Source: CAD feature listing. Evaluate the final solid. Frame: model axes, mm. Face numbers are marked on the shaded views. A direction names the side the tool comes from. Round coordinates to 2 decimals unless told otherwise and drop trailing zeros. Write each loop counter-clockwise with the first axis right and the second up, starting at its lowest first coordinate (ties: lowest second). Pieces come first, ordered by that corner, then holes.
```python
from build123d import *

# Parameters (mm, degrees)
MAIN_BODY_DEPTH      = 15
HOLES_DEPTH          = 84.815273071
HEX_NUT_RECESS_DEPTH = 3


with BuildPart() as part:
    # Schizzo2 → Main Body (new, symmetric)
    with BuildSketch(Plane(origin=(0, 0, 0), x_dir=(1, 0, 0), z_dir=(0, 1, 0))):
        with BuildLine():
            Line((0, 0), (0, 20))
            Line((0, 20), (24.437059837, 20))
            Line((24.437059837, 20), (24.437059837, 10.75))
            Line((24.437059837, 10.75), (14.437059837, 10.75))
            ThreePointArc((14.437059837, 10.75), (5.5, 10), (14.437059837, 9.25))
            Line((14.437059837, 9.25), (80, 9.25))
            Line((80, 9.25), (80, 0))
            Line((80, 0), (0, 0))
        make_face()
    extrude(amount=MAIN_BODY_DEPTH, both=True)

    # Schizzo3 → Holes (cut, through all)
    with BuildSketch(Plane(origin=(0, 0, -20), x_dir=(-1, 0, 0), z_dir=(0, 0, -1))):
        with BuildLine():
            Line((-20.447422808, -5.75), (-18.426696866, -5.75))
            Line((-18.426696866, -5.75), (-17.921515381, -6.625))
            ThreePointArc((-17.921515381, -6.625), (-19.437059837, -9.25), (-20.952604294, -6.625))
            Line((-20.952604294, -6.625), (-20.447422808, -5.75))
        make_face()
        with BuildLine():
            Line((-20.447422808, 9.25), (-18.426696866, 9.25))
            Line((-18.426696866, 9.25), (-17.921515381, 8.375))
            ThreePointArc((-17.921515381, 8.375), (-19.437059837, 5.75), (-20.952604294, 8.375))
            Line((-20.952604294, 8.375), (-20.447422808, 9.25))
        make_face()
    extrude(amount=-HOLES_DEPTH, mode=Mode.SUBTRACT)

    # Schizzo4 → Hex nut recess (cut)
    with BuildSketch(Plane.XY):
        Polygon((19.437059837, 11.25277675), (16.187059837, 9.376388375), (16.187059837, 5.623611625), (19.437059837, 3.74722325), (22.687059837, 5.623611625), (22.687059837, 9.376388375), align=None)
        Polygon((19.437059837, -3.74722325), (16.187059837, -5.623611625), (16.187059837, -9.376388375), (19.437059837, -11.25277675), (22.687059837, -9.376388375), (22.687059837, -5.623611625), align=None)
    extrude(amount=-HEX_NUT_RECESS_DEPTH, mode=Mode.SUBTRACT)


solid = part.part
```
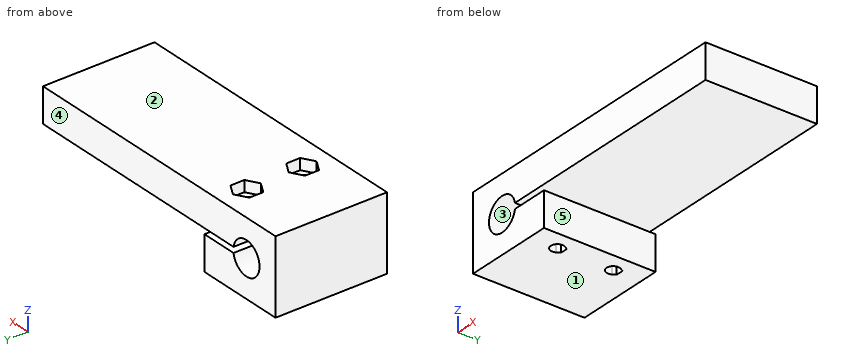
Q1. Section query C-C, the plane y = 7.5. Output: boundary loops of the cut face in (x, z), and give its area (3 significant figures).
Q2. Pin query (flat end, axial travel): P1, Ø5, axis at y = 10, z = -5, coming from the -X side; P2, Ø1.5, axis at x = 52.5, y = -7.5, coming from the -Z side; P3, Ø4.5, axis at y = -6.5, z = -16.5, coming from the +X side; P4, Ø3, axis at x = 19.5, y = 9, coming from the +Z side. Return the tip coordinate at first contact, or that it passes through.
Q3. Section query A-A, the plane z = -7.5. Output: boundary loops of the cut face in (x, y) (3 decimals), and give its area (3 significant figures).
Q4. Line query: line 1 (Z direction, x = 21.5, y = -5.5); line 2 (X direction, y = 7.5, z = -5); line 3 (X direction, y = 7.5, z = -7.25). Output: solid intervals per line, ascending.
Q5. Mould query, pull axis Z, two halves, no side actions, for the marked faces 1, 2 and 3. Classes: pulls with the +Z half, pulls with the -Z half, needs draft (parallel to the pull), parting line crosses it, or undercut.
Q6. Set-up query: the marked faces 4 and 5. Return all of +Z, -Z, +X, -X, +Y, -Y with unobstructed straight access to the full face (end or side cutting, diameter ignored); none if empty.
Q7. Section query D-D, the plane z = -17.5. Output: boundary loops of the cut face in (x, y) (3 decimals), and give its area (3 significant figures).
Q8. Section query B-B, the plane x = 10. Output: boundary loops of the cut face in (y, z).
Filled in:
1. outline: (0, -20) - (17.69, -20) - (17.69, -10.75) - (14.44, -10.75) arc R4.5 cw (long way) to (14.44, -9.25) - (17.69, -9.25) - (17.69, -3) - (16.19, -3) - (16.19, 0) - (0, 0) - close; (21.19, -20) - (24.44, -20) - (24.44, -10.75) - (21.19, -10.75) - close; (21.19, -9.25) - (80, -9.25) - (80, 0) - (22.69, 0) - (22.69, -3) - (21.19, -3) - close
1. area: 850 mm2
2. P1: stops at x = 0
2. P2: stops at z = -9.25
2. P3: stops at x = 24.44
2. P4: stops at z = -3
3. outline: (0, -15) - (6.258, -15) - (6.258, 15) - (0, 15) - close; (13.742, -15) - (80, -15) - (80, 15) - (13.742, 15) - close; hole (17.922, -6.625) arc R1.75 ccw (long way) to (20.953, -6.625) - (20.447, -5.75) - (18.427, -5.75) - close; hole (17.922, 8.375) arc R1.75 ccw (long way) to (20.953, 8.375) - (20.447, 9.25) - (18.427, 9.25) - close
3. area: 2,160 mm2
4. line 1: z = -20 to -10.75, -9.25 to -3
4. line 2: x = 0 to 17.69, 21.19 to 80
4. line 3: x = 0 to 6.44, 13.56 to 17.69, 21.19 to 80
5. face 1: pulls with the -Z half
5. face 2: pulls with the +Z half
5. face 3: undercut
6. face 4: +Z, -Z, +X, -X, +Y
6. face 5: -Z, +X, +Y, -Y
7. outline: (0, -15) - (24.437, -15) - (24.437, 15) - (0, 15) - close; hole (17.922, -6.625) arc R1.75 ccw (long way) to (20.953, -6.625) - (20.447, -5.75) - (18.427, -5.75) - close; hole (17.922, 8.375) arc R1.75 ccw (long way) to (20.953, 8.375) - (20.447, 9.25) - (18.427, 9.25) - close
7. area: 713 mm2
8. outline: (-15, -20) - (15, -20) - (15, -14.5) - (-15, -14.5) - close; (-15, -5.5) - (15, -5.5) - (15, 0) - (-15, 0) - close
